The drawing under review shows one solid part. Ordinate dimensions are in mm from its lowest x, y, z. A direction names the side the tool comes from. Round coordinates to 2 decimals unless told otherwise and drop trailing zeros. Write each loop counter-clockwise with the first axis right and the second up, starting at its lowest first coordinate (ties: lowest second). Pieces come first, ordered by that corner, then holes. Notation, with made-up numbers: M -34,80.5 L -10,80.5 A23 ccw -10,111.5 Z; hole C 37,24.25 d11. An arc over 180 degrees is marked long. One line per item, written item: value. Start each with the question number.
1) Take a section at B-B, the plane x = 6.5. Write out the cut boundary in (y, z).
2) Take a section at A-A, the plane y = 7.25. Write out the cut boundary in (x, z).
3) Wall thickness on probe 1 along Z at (x, y) = (5, 5.5); probe 2 along X at (y, z) = (4.25, 11); probe 3 along Y at (x, z) = (5, 28) (1 decimal): over which ranges is each line inside the solid? List them lowest first.
4) For P1, Ø3, axis at x = 6, z = 31, coming from the +Y side; P2, Ø3, axis at x = 3, y = 2, coming from the -Z side; P3, Ø4, axis at x = 2, z = 12, coming from the +Y side; P4, Ø3, axis at x = 5, z = 19.5, coming from the -Y side, all flat-tipped, find the tip position at first contact; note any pin that passes through.
5) Take a section at C-C, the plane z = 33. Write out the cut boundary in (x, y), and give its area (3 significant figures).
6) Tool access review of the marked faces 1 and 2: name each direction out of +Z, -Z, +X, -X, +Y, -Y from which nothing blocks a thin tool from reaching the whole face with its end or side.
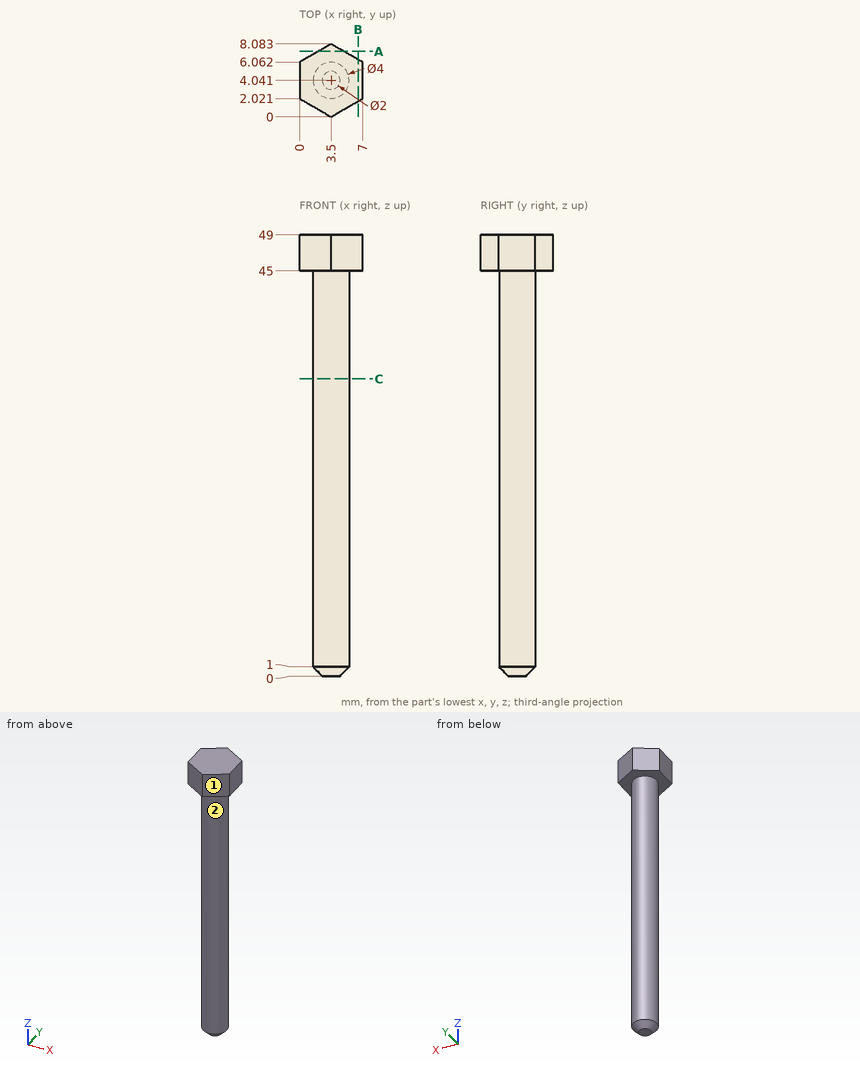
Checked values:
1. outline: M 1.73,45 L 6.35,45 L 6.35,49 L 1.73,49 Z
2. outline: M 2.06,45 L 4.94,45 L 4.94,49 L 2.06,49 Z
3. probe 1: z = 45 to 49
3. probe 2: x = 1.51 to 5.49
3. probe 3: y = 2.7 to 5.4
4. P1: stops at y = 5.77
4. P2: stops at z = 0
4. P3: stops at y = 6.04
4. P4: stops at y = 2.04
5. outline: C 3.5,4.04 d4
5. area: 12.6 mm2
6. face 1: +Z, -Z, +X, -Y
6. face 2: -Z
